Could you check a few things on this model? Use its own coordinates, in mm. Face numbers are marked on the shaded views. A direction names the side the tool comes from. Round coordinates to 2 decimals unless told otherwise and drop trailing zeros. Loops run counter-clockwise (first coordinate to the right, second up) from the corner with the lowest first, then second, coordinate; pieces in that order, holes last. Notation, with made-up numbers: (36, -12) - (41, -12) arc R23 cw to (41, 3) - close; hole circle Ø4 at (28, 40.25). An arc over 180 degrees is marked (long way). Use one line per item in the form item = value.
```python
from build123d import *

# Parameters (mm, degrees)
SKETCH1_W           = 76.2
SKETCH1_H           = 50.8
BOSS_EXTRUDE1_DEPTH = 19.05
SKETCH2_W           = 34.925
SKETCH2_H           = 44.45
CUT_EXTRUDE1_DEPTH  = 16.51
SKETCH4_R           = 1.016
CUT_EXTRUDE4_DEPTH  = 5.08
SKETCH6_R           = 1.016
CUT_EXTRUDE6_DEPTH  = 94.057294717


with BuildPart() as part:
    # Sketch1 → Boss-Extrude1 (new body)
    with BuildSketch(Plane.XY):
        with Locations((38.1, 25.4)):
            Rectangle(SKETCH1_W, SKETCH1_H)
    extrude(amount=BOSS_EXTRUDE1_DEPTH)

    # Sketch2 → Cut-Extrude1 (cut)
    with BuildSketch(Plane.XY.offset(19.05)):
        with Locations((55.5625, 25.4)):
            Rectangle(SKETCH2_W, SKETCH2_H)
        with Locations((20.6375, 25.4)):
            Rectangle(SKETCH2_W, SKETCH2_H)
    extrude(amount=-CUT_EXTRUDE1_DEPTH, mode=Mode.SUBTRACT)

    # Sketch4 → Cut-Extrude4 (cut)
    with BuildSketch(Plane.XY.offset(19.05)):
        with Locations((1.5875, 25.4)):
            Circle(SKETCH4_R)
        with Locations((38.1, 49.2125)):
            Circle(SKETCH4_R)
        with Locations((74.6125, 25.4)):
            Circle(SKETCH4_R)
        with Locations((38.1, 1.5875)):
            Circle(SKETCH4_R)
    extrude(amount=-CUT_EXTRUDE4_DEPTH, mode=Mode.SUBTRACT)

    # Sketch6 → Cut-Extrude6 (cut, through all)
    with BuildSketch(Plane.XY.offset(2.54)):
        with Locations((26.310023895, 25.4)):
            Circle(SKETCH6_R)
        with Locations((44.090023895, 25.4)):
            Circle(SKETCH6_R)
    extrude(amount=-CUT_EXTRUDE6_DEPTH, mode=Mode.SUBTRACT)


solid = part.part
```
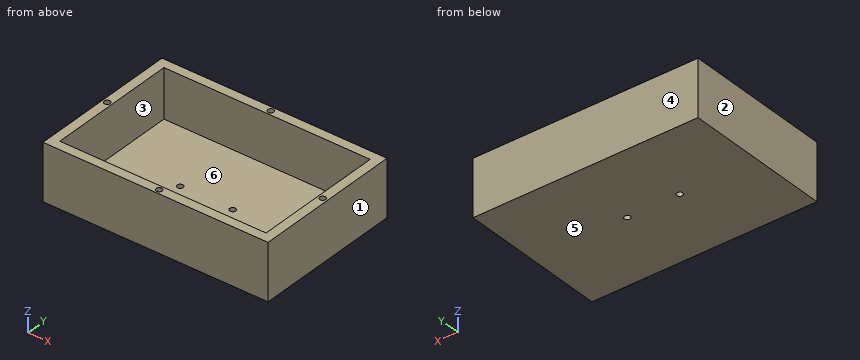
1. If we section it at D-D, the plane x = 21: Write out the boundary of the cut face in (y, z) (3 decimals), plus the area to 3 significant figures.
Solution:
outline = (0, 0) - (50.8, 0) - (50.8, 19.05) - (47.625, 19.05) - (47.625, 2.54) - (3.175, 2.54) - (3.175, 19.05) - (0, 19.05) - close
area = 234 mm^2
2. If we section it at C-C, the plane y = 9: Write out the boundary of the cut face in (x, z) (3 decimals), plus the area to 3 significant figures.
Solution:
outline = (0, 0) - (76.2, 0) - (76.2, 19.05) - (73.025, 19.05) - (73.025, 2.54) - (3.175, 2.54) - (3.175, 19.05) - (0, 19.05) - close
area = 298 mm^2
3. If we section it at A-A, the plane y = 25.4: Count the separate pieces of the cut face and the enclosed holes in it, plus the area to 3 significant figures.
Solution:
separate_pieces = 3
enclosed_holes = 0
area = 267 mm^2
4. On a 3-axis mill with a long thin cutter (end or side, diameter ignored), from which of +Z, -Z, +X, -X, +Y, -Y can I reach the whole of each face in a straight line? I mean the marked faces 5 and 6. Say none if no direction works.
Solution:
face_5 = -Z, +X, -X, +Y, -Y
face_6 = +Z
5. If we section it at B-B, the plane z = 10.5: Write out the boundary of the cut face in (x, y) (3 decimals), plus the area to 3 significant figures.
Solution:
outline = (0, 0) - (76.2, 0) - (76.2, 50.8) - (0, 50.8) - close; hole (3.175, 3.175) - (73.025, 3.175) - (73.025, 47.625) - (3.175, 47.625) - close
area = 766 mm^2
6. Please list where these lines run through material, in increasing order: line 1 along Y through (x, z) = (38.1, 16.2) (1 decimal); line 2 along Y through (x, z) = (24, 15) (3 decimals); line 3 along X through (y, z) = (25, 12) (3 decimals).
Solution:
line_1 = 0 to 0.6, 2.6 to 3.2, 47.6 to 48.2, 50.2 to 50.8
line_2 = 0 to 3.175, 47.625 to 50.8
line_3 = 0 to 3.175, 73.025 to 76.2
7. We'd pull the mould along X, two halves only. Please class the marked faces 1, 2, 3 and 4: +X half, -X half, draft (parallel to the pull), parting line (faces both ways), or undercut.
Solution:
face_1 = +X half
face_2 = -X half
face_3 = undercut
face_4 = draft
8. For P1, Ø1, axis at x = 21.5, y = 17.5, coming from the -Z side; P2, Ø1.6, axis at x = 26.31, y = 25.4, coming from the -Z side; P3, Ø1.5, axis at x = 18.5, y = 10.5, coming from the +Z side; P4, Ø0.6, axis at x = 74, y = 25.5, coming from the +Z side, each with a flat end and sliding along its axis, tell me the tip position at first contact or that it passes through.
Solution:
P1 = 0
P2 = through
P3 = 2.54
P4 = 13.97
